from build123d import *

# Parameters (mm, degrees)
F0_W     = 3
F0_H     = 6
F1_DEPTH = 8
F3_D     = 4
F3_DEPTH = 10
F4_R     = 3
F5_R     = 2


with BuildPart() as f1:
    # F0 (on Top) → F1 (new body)
    with BuildSketch(Plane.XY):
        Polygon((0, -78), (0, 0), (72, 0), (72, 3), (-3, 3), (-3, -81), (9, -81), (9, -78), (6, -78), align=None)
        with Locations((7.5, -75)):
            Rectangle(F0_W, F0_H)
    extrude(amount=F1_DEPTH)

    # F3
    with Locations(Plane(origin=(0, 3, 0), x_dir=(-1, 0, 0), z_dir=(0, 1, 0))):
        with Locations((-64, 4)):
            Hole(F3_D / 2, depth=F3_DEPTH)

    # F4
    f4_edges = [f1.edges().sort_by_distance(p)[0] for p in [
        (-3, -81, 4),
        (-3, 3, 4),
        (9, -81, 4),
    ]]
    fillet(f4_edges, radius=F4_R)

    # F5
    f5_edges = [f1.edges().sort_by_distance(p)[0] for p in [
        (6, -78, 4),
        (0, -78, 4),
        (0, 0, 4),
    ]]
    fillet(f5_edges, radius=F5_R)


solid = f1.part
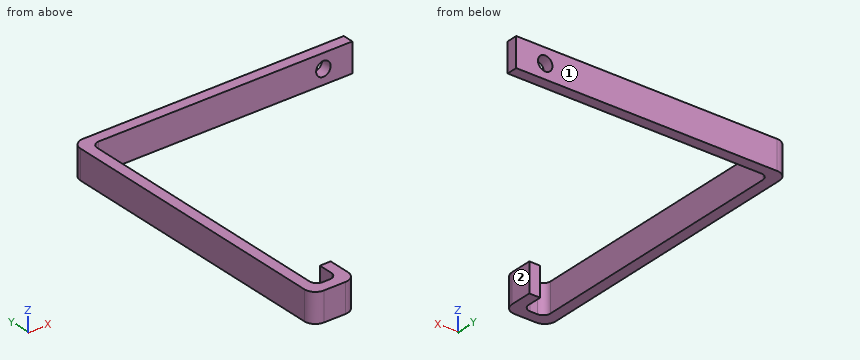
Verification items for the finished model (mm, model axes). Face numbers are marked on the shaded views. A direction names the side the tool comes from. Coordinates: 2 decimals unless noted, no trailing zeros. Order: outer loops, then holes, each group sorted by start corner. A loop starts at its lowest first (then second) coordinate and runs counter-clockwise, first axis right, second up. Notation, with made-up numbers: M 88.5,65 L 116.5,65 A22 ccw 116.5,81 Z; hole C -34,78 d3. An arc over 180 degrees is marked long. One line per item, written item: value. Start each with the question number.
Item 1: Sectioned sample at B-B on x = 64. Record the cut outline in (y, z).
Item 2: Thickness scan on probe 1 along Z at (x, y) = (64, 1.1); probe 2 along X at (y, z) = (-67, 2); probe 3 along Y at (x, z) = (50, 0.5). Record the ranges inside material, lowest first.
Item 3: Depth check by flat-ended pin: P1, Ø4, axis at y = -50.5, z = 3, coming from the +X side; P2, Ø1.8, axis at y = -74, z = 2, coming from the +X side; P3, Ø2.5, axis at x = 39, z = 5, coming from the -Y side. Enter the tip coordinate at first touch or a pass-through.
Item 4: Sectioned sample at A-A on z = 4. Record the cut outline in (x, y), then the cut area to 3 significant figures.
Item 5: Sectioned sample at C-C on y = -5. Record the cut outline in (x, z).
Item 6: Access from +Z, -Z, +X, -X, +Y, -Y to the whole of each face (thin tool, end or side, straight path). Record for the marked faces 1 and 2.
Calculated:
1. outline: M 0,0 L 3,0 L 3,2 L 0,2 Z; M 0,6 L 3,6 L 3,8 L 0,8 Z
2. probe 1: 0 to 2, 6 to 8
2. probe 2: -3 to 0
2. probe 3: 0 to 3
3. P1: x = 0
3. P2: x = 9
3. P3: y = 0
4. outline: M -3,-78 A3 ccw 0,-81 L 6,-81 A3 ccw 9,-78 L 9,-72 L 6,-72 L 6,-76 A2 cw 4,-78 L 2,-78 A2 cw 0,-76 L 0,-2 A2 cw 2,0 L 62,0 L 62,3 L 0,3 A3 ccw -3,0 Z; M 66,0 L 72,0 L 72,3 L 66,3 Z
4. area: 498 mm^2
5. outline: M -3,0 L 0,0 L 0,8 L -3,8 Z
6. face 1: +Z, -Z, +X, -X, +Y
6. face 2: +Z, -Z, +X, -Y
